```python
from build123d import *

# Parameters (mm, degrees)
BOSS_EXTRUDE1_DEPTH = 101.6
SKETCH3_W           = 20.32
SKETCH3_H           = 1346.2
CUT_EXTRUDE1_DEPTH  = 10.16
SKETCH4_W           = 20.32
SKETCH4_H           = 1346.2
CUT_EXTRUDE2_DEPTH  = 10.16


with BuildPart() as part:
    # Sketch2 → Boss-Extrude1 (new body)
    with BuildSketch(Plane.XY):
        Polygon((-520.7, 711.2), (495.299974685, 710.973195751), (520.7, -711.2), (-520.7, -711.2), align=None)
        Polygon((-482.6, 673.091493891), (457.874215728, 672.881549449), (481.913457595, -673.1), (-482.6, -673.1), align=None, mode=Mode.SUBTRACT)
    extrude(amount=BOSS_EXTRUDE1_DEPTH)

    # Sketch3 → Cut-Extrude1 (cut)
    with BuildSketch(Plane(origin=(469.742047624, 8.389596947, 0), x_dir=(0, 0, 1), z_dir=(-0.9998405481942395, -0.01785716065455791, 0))):
        with Locations((50.8, -8.500177591)):
            Rectangle(SKETCH3_W, SKETCH3_H)
    extrude(amount=-CUT_EXTRUDE1_DEPTH, mode=Mode.SUBTRACT)

    # Sketch4 → Cut-Extrude2 (cut)
    with BuildSketch(Plane(origin=(-482.6, 0, 0), x_dir=(0, 0, -1), z_dir=(1, 0, 0))):
        with Locations((-50.8, -0.004253054)):
            Rectangle(SKETCH4_W, SKETCH4_H)
    extrude(amount=-CUT_EXTRUDE2_DEPTH, mode=Mode.SUBTRACT)


solid = part.part
```
For this review, take the finished solid that the model builds, in its own axes (mm). A direction names the side the tool comes from. Round coordinates to 2 decimals unless told otherwise and drop trailing zeros. Order: outer loops, then holes, each group sorted by start corner. A loop starts at its lowest first (then second) coordinate and runs counter-clockwise, first axis right, second up.
Q1. We need section C-C, the plane x = 411. Give the boundary of the cut face in (y, z).
Findings below:
outline: (-711.2, 0) - (-673.1, 0) - (-673.1, 101.6) - (-711.2, 101.6) - close; (672.89, 0) - (710.99, 0) - (710.99, 101.6) - (672.89, 101.6) - close
Q2. Machinability: for faces 4 (the flat face through (-482.6, -9, 81)), 5 (the flat face through (475, -9, 60.96)), 6 (the flat face through (7, -711.2, 50)), which of the approach directions +Z, -Z, +X, -X, +Y, -Y give a long, thin tool a straight path to every point of the face, cutting with its end or side? Answer none if there is none.
Findings below:
face 4: +Z, -Z
face 5: none
face 6: +Z, -Z, +X, -X, -Y
Q3. We need section B-B, the plane y = 476.5. Give the boundary of the cut face in (x, z).
Findings below:
outline: (-520.7, 0) - (-482.6, 0) - (-482.6, 40.64) - (-492.76, 40.64) - (-492.76, 60.96) - (-482.6, 60.96) - (-482.6, 101.6) - (-520.7, 101.6) - close; (461.38, 0) - (499.49, 0) - (499.49, 101.6) - (461.38, 101.6) - (461.38, 60.96) - (471.54, 60.96) - (471.54, 40.64) - (461.38, 40.64) - close
Q4. Mouldability with a two-part tool opening along X and no side actions: class faces 1 (the flat face through (6, -673.1, 50)), 2 (the flat face through (-520.7, -10, 50)), 3 (the flat face through (-499, 3, 101.6)) as pulls with the +X half, pulls with the -X half, needs draft (parallel to the pull), parting line crosses it, or undercut.
Findings below:
face 1: undercut
face 2: pulls with the -X half
face 3: needs draft
Q5. We need section A-A, the plane z = 26.5. Give the boundary of the cut face in (x, y).
Findings below:
outline: (-520.7, -711.2) - (520.7, -711.2) - (495.3, 710.97) - (-520.7, 711.2) - close; hole (-482.6, -673.1) - (481.91, -673.1) - (457.87, 672.88) - (-482.6, 673.09) - close
Q6. Wall thickness on line 1 (Y direction, x = 432.5, z = 50.5); line 2 (Y direction, x = 64, z = 68.5); line 3 (X direction, y = 495, z = 74.5): over which ranges is each line inside the solid? List them lowest first.
Findings below:
line 1: y = -711.2 to -673.1, 672.89 to 710.99
line 2: y = -711.2 to -673.1, 672.97 to 711.07
line 3: x = -520.7 to -482.6, 461.05 to 499.16
Q7. Insertion check: P1, Ø16.5, axis at y = 161, z = 47, coming from the +X side; P2, Ø5, axis at x = -486, z = 49.5, coming from the +Y side; P3, Ø6, axis at y = 393.5, z = 29, coming from the +X side. Each pin has a flat end and moves straight along its axis. Give the tip position at first contact, or say it passes through.
Findings below:
P1: stops at x = 505.27
P2: stops at y = 711.19
P3: stops at x = 501.02
